Geometry: final body of the model. Coordinates: model frame, mm. A direction names the side the tool comes from. Give positions to 0.01 mm unless a question says otherwise; leave off trailing zeros. Write each loop counter-clockwise with the first axis right and the second up, starting at its lowest first coordinate (ties: lowest second). Pieces come first, ordered by that corner, then holes. Notation, with made-up numbers: M -5.5,-31 L 31.5,-31 A20 cw 31.5,-25 Z; hole C 21,84 d7. An arc over 180 degrees is marked long. One line per question, with ' | ' between items.
from build123d import *

# Parameters (mm, degrees)
ESQUISSE1_W             = 232.41
ESQUISSE1_H             = 5.08
EXTRU_MINCE1_DEPTH      = 19.05
EXTRU_MINCE2_DEPTH      = 26.67
BOSS_EXTRU_2_DEPTH      = 7.62
ESQUISSE2_W             = 29.21
ESQUISSE2_H             = 57.15
ENL_V_MAT_EXTRU_1_DEPTH = 10.16
ENL_V_MAT_EXTRU_2_REACH = 123.325
ESQUISSE7_R             = 1.65
ESQUISSE8_R             = 10.16
ENL_V_MAT_EXTRU_3_DEPTH = 122.324888729
ESQUISSE9_W             = 10.16
ESQUISSE9_H             = 10.16
BOSS_EXTRU_1_DEPTH      = 2.54
D_GAGEMENT_61_D         = 3.7973
D_GAGEMENT_61_DEPTH     = 2.54
ESQUISSE12_W            = 10.16
ESQUISSE12_H            = 81.28
ENL_V_MAT_EXTRU_4_DEPTH = 3.81
ENL_V_START             = -8.89
ENL_V_MAT_EXTRU_5_DEPTH = 8.89
D_GAGEMENT_62_D         = 3.7973


with BuildPart() as part:
    # Esquisse1 → Extru.-Mince1 (new, symmetric)
    with BuildSketch(Plane(origin=(0, 0, 0), x_dir=(0, 0, -1), z_dir=(1, 0, 0))):
        with Locations((0, 46.628736397)):
            Rectangle(ESQUISSE1_W, ESQUISSE1_H)
    extrude(amount=EXTRU_MINCE1_DEPTH, both=True)

    # Esquisse6 → Extru.-Mince2 (add)
    with BuildSketch(Plane(origin=(0, 49.168736397, 0), x_dir=(1, 0, 0), z_dir=(0, 1, 0))):
        with BuildLine():
            Line((-19.0246, -24.3459), (-19.0246, 24.3459))
            ThreePointArc((-19.0246, 24.3459), (0, 43.3705), (19.0246, 24.3459))
            Line((19.0246, 24.3459), (19.0246, -24.3459))
            ThreePointArc((19.0246, -24.3459), (0, -43.3705), (-19.0246, -24.3459))
        make_face()
        with BuildLine():
            Line((-16.4846, -24.3459), (-16.4846, 24.3459))
            ThreePointArc((-16.4846, 24.3459), (0, 40.8305), (16.4846, 24.3459))
            Line((16.4846, 24.3459), (16.4846, -24.3459))
            ThreePointArc((16.4846, -24.3459), (0, -40.8305), (-16.4846, -24.3459))
        make_face(mode=Mode.SUBTRACT)
    extrude(amount=EXTRU_MINCE2_DEPTH)

    # Esquisse13 → Boss.-Extru.2 (add)
    with BuildSketch(Plane(origin=(0, 49.168736397, 0), x_dir=(1, 0, 0), z_dir=(0, 1, 0))):
        with BuildLine():
            Line((-16.4846, 24.3459), (-16.4846, -24.3459))
            ThreePointArc((-16.4846, -24.3459), (0, -40.8305), (16.4846, -24.3459))
            Line((16.4846, -24.3459), (16.4846, 24.3459))
            ThreePointArc((16.4846, 24.3459), (0, 40.8305), (-16.4846, 24.3459))
        make_face()
    extrude(amount=BOSS_EXTRU_2_DEPTH)

    # Esquisse2 → Enlèv. mat.-Extru.1 (cut)
    with BuildSketch(Plane(origin=(0, 56.788736397, 0), x_dir=(1, 0, 0), z_dir=(0, 1, 0))):
        Rectangle(ESQUISSE2_W, ESQUISSE2_H)
    extrude(amount=-ENL_V_MAT_EXTRU_1_DEPTH, mode=Mode.SUBTRACT)

    # Esquisse7 → Enlèv. mat.-Extru.2 (cut, up to next)
    with BuildSketch(Plane(origin=(0, 46.628736397, 0), x_dir=(1, 0, 0), z_dir=(0, 1, 0)), mode=Mode.PRIVATE) as enl_v_mat_extru_2_sk1:
        with Locations(Location((-9.525, 9.525, 0), (0, 0, 270))):
            Circle(ESQUISSE7_R)
    enl_v_mat_extru_2_tool1 = extrude(enl_v_mat_extru_2_sk1.sketch, amount=-ENL_V_MAT_EXTRU_2_REACH, mode=Mode.PRIVATE) & part.part
    # Esquisse7 → Enlèv. mat.-Extru.2 (cut, up to next)
    with BuildSketch(Plane(origin=(0, 46.628736397, 0), x_dir=(1, 0, 0), z_dir=(0, 1, 0)), mode=Mode.PRIVATE) as enl_v_mat_extru_2_sk2:
        with Locations(Location((9.525, 9.525, 0), (0, 0, 270))):
            Circle(ESQUISSE7_R)
    enl_v_mat_extru_2_tool2 = extrude(enl_v_mat_extru_2_sk2.sketch, amount=-ENL_V_MAT_EXTRU_2_REACH, mode=Mode.PRIVATE) & part.part
    # Esquisse7 → Enlèv. mat.-Extru.2 (cut, up to next)
    with BuildSketch(Plane(origin=(0, 46.628736397, 0), x_dir=(1, 0, 0), z_dir=(0, 1, 0)), mode=Mode.PRIVATE) as enl_v_mat_extru_2_sk3:
        with Locations(Location((9.525, -9.525, 0), (0, 0, 270))):
            Circle(ESQUISSE7_R)
    enl_v_mat_extru_2_tool3 = extrude(enl_v_mat_extru_2_sk3.sketch, amount=-ENL_V_MAT_EXTRU_2_REACH, mode=Mode.PRIVATE) & part.part
    # Esquisse7 → Enlèv. mat.-Extru.2 (cut, up to next)
    with BuildSketch(Plane(origin=(0, 46.628736397, 0), x_dir=(1, 0, 0), z_dir=(0, 1, 0)), mode=Mode.PRIVATE) as enl_v_mat_extru_2_sk4:
        with Locations(Location((-9.525, -9.525, 0), (0, 0, 270))):
            Circle(ESQUISSE7_R)
    enl_v_mat_extru_2_tool4 = extrude(enl_v_mat_extru_2_sk4.sketch, amount=-ENL_V_MAT_EXTRU_2_REACH, mode=Mode.PRIVATE) & part.part
    add(enl_v_mat_extru_2_tool1.solids().sort_by_distance((-9.525, 46.628736, -9.525))[0], mode=Mode.SUBTRACT)
    add(enl_v_mat_extru_2_tool2.solids().sort_by_distance((9.525, 46.628736, -9.525))[0], mode=Mode.SUBTRACT)
    add(enl_v_mat_extru_2_tool3.solids().sort_by_distance((9.525, 46.628736, 9.525))[0], mode=Mode.SUBTRACT)
    add(enl_v_mat_extru_2_tool4.solids().sort_by_distance((-9.525, 46.628736, 9.525))[0], mode=Mode.SUBTRACT)

    # Esquisse8 → Enlèv. mat.-Extru.3 (cut, through all)
    with BuildSketch(Plane(origin=(0, 46.628736397, 0), x_dir=(1, 0, 0), z_dir=(0, 1, 0))):
        with Locations(Location((0, 0, 0), (0, 0, 270))):
            Circle(ESQUISSE8_R)
    extrude(amount=-ENL_V_MAT_EXTRU_3_DEPTH, mode=Mode.SUBTRACT)

    # Esquisse9 → Boss.-Extru.1 (add)
    with BuildSketch(Plane(origin=(0, 75.838736397, 0), x_dir=(1, 0, 0), z_dir=(0, 1, 0))):
        with Locations((0, 45.9105)):
            Rectangle(ESQUISSE9_W, ESQUISSE9_H)
    boss_extru_1 = extrude(amount=-BOSS_EXTRU_1_DEPTH)

    # Dégagement #61
    with Locations(Plane(origin=(0, 75.838736397, 0), x_dir=(1, 0, 0), z_dir=(0, 1, 0))):
        with Locations((0, 46.835110673)):
            d_gagement_61 = Hole(D_GAGEMENT_61_D / 2, depth=D_GAGEMENT_61_DEPTH)

    # Symétrie1: Boss.-Extru.1, Dégagement #61 across plane
    add(boss_extru_1.mirror(Plane.XY))
    add(d_gagement_61.mirror(Plane.XY), mode=Mode.SUBTRACT)

    # Esquisse12 → Enlèv. mat.-Extru.4 (cut)
    with BuildSketch(Plane(origin=(0, 44.088736397, 0), x_dir=(1, 0, 0), z_dir=(0, 1, 0))):
        with Locations((0, -69.215)):
            Rectangle(ESQUISSE12_W, ESQUISSE12_H)
    extrude(amount=ENL_V_MAT_EXTRU_4_DEPTH, mode=Mode.SUBTRACT)

    # Esquisse14 → Enlèv. mat.-Extru.5 (cut)
    with BuildSketch(Plane(origin=(0, 56.788736397, 0), x_dir=(1, 0, 0), z_dir=(0, 1, 0)).offset(ENL_V_START)):
        with BuildLine():
            Line((-5.08, -28.575), (5.08, -28.575))
            Line((5.08, -28.575), (5.08, -40.028235195))
            ThreePointArc((5.08, -40.028235195), (0, -40.8305), (-5.08, -40.028235195))
            Line((-5.08, -40.028235195), (-5.08, -28.575))
        make_face()
    extrude(amount=ENL_V_MAT_EXTRU_5_DEPTH, mode=Mode.SUBTRACT)

    # Dégagement #62 (through all)
    with Locations(Plane(origin=(0, 49.168736397, 0), x_dir=(1, 0, 0), z_dir=(0, 1, 0))):
        with Locations((-9.525, 100.965), (9.525, 100.965), (9.525, -100.965), (-9.525, -100.965)):
            Hole(D_GAGEMENT_62_D / 2)


solid = part.part
(1) Cut plane A-A, the plane z = 0. Return loops of the section in (x, y) (3 decimals).
Working result:
outline: M -19.05,44.089 L -10.16,44.089 L -10.16,46.629 L -14.605,46.629 L -14.605,56.789 L -16.485,56.789 L -16.485,75.839 L -19.025,75.839 L -19.025,49.169 L -19.05,49.169 Z; M 10.16,44.089 L 19.05,44.089 L 19.05,49.169 L 19.025,49.169 L 19.025,75.839 L 16.485,75.839 L 16.485,56.789 L 14.605,56.789 L 14.605,46.629 L 10.16,46.629 Z
(2) Cut plane B-B, the plane y = 54.5. Return loops of the section in (x, z) (3 decimals).
Working result:
outline: M -19.025,-24.346 A19.025 ccw 19.025,-24.346 L 19.025,24.346 A19.025 ccw -19.025,24.346 Z; hole M -14.605,-28.575 L 14.605,-28.575 L 14.605,28.575 L 5.08,28.575 L 5.08,40.028 A16.485 ccw -5.08,40.028 L -5.08,28.575 L -14.605,28.575 Z
(3) Material intervals for L1, parallel to Z at x = 0, y = 75; L2, parallel to X at y = 66.5, z = 20.5; L3, parallel to Y at x = 8, z = 86, sorted ascending. Write a range as [from, to].
Working result:
L1: z = [-50.99, -48.73], [-44.94, -40.83], [40.83, 44.94], [48.73, 50.99] | L2: x = [-19.02, -16.48], [16.48, 19.02] | L3: y = [44.09, 49.17]
(4) Cut plane D-D, the plane z = -81.5. Return loops of the section in (x, y), then the cut area to 3 significant figures.
Working result:
outline: M -19.05,44.09 L 19.05,44.09 L 19.05,49.17 L -19.05,49.17 Z | area: 194 mm^2
(5) Draft query along Z for faces 4 (the face through (0, 47, -116.205)), 5 (the face through (-0.362, 66.18, -40.827)), 6 (the face through (13, 44.089, 2)). Return one class per face: released by +Z, released by -Z, zero draft, split by the parting line, or undercut.
Working result:
face 4: released by -Z | face 5: undercut | face 6: zero draft
(6) Cut plane C-C, the plane z = 68.5. Return loops of the section in (x, y).
Working result:
outline: M -19.05,44.09 L -5.08,44.09 L -5.08,47.9 L 5.08,47.9 L 5.08,44.09 L 19.05,44.09 L 19.05,49.17 L -19.05,49.17 Z
(7) Set-up query: faces 1 (the face through (-14.605, 52, 0)), 2 (the face through (-5.08, 47.5, 60.8)), 3 (the face through (8.504, 46.593, 99.364)). Return all of +Z, -Z, +X, -X, +Y, -Y with unobstructed straight access to the full face (end or side cutting, diameter ignored); none if empty.
Working result:
face 1: +Y | face 2: -Y | face 3: +Y, -Y
(8) First-contact query: P1, Ø3, axis at x = 7.5, y = 51.5, coming from the -Z side; P2, Ø11, axis at x = -4.5, y = 51.5, coming from the +Z side (3 decimals); P3, Ø2, axis at x = 15, z = 44, coming from the +Y side; P4, Ø3, axis at x = -2, y = 74.5, coming from the -Z side. Flat tips, straight axial feed; report the tip coordinate or a pass-through.
Working result:
P1: stops at z = -42.4 | P2: stops at z = 116.205 | P3: stops at y = 49.17 | P4: stops at z = -50.99
